The listing builds one solid part. Answer for the finished solid, in the listing's coordinates (mm). Face numbers are marked on the shaded views. A direction names the side the tool comes from. Round coordinates to 2 decimals unless told otherwise and drop trailing zeros. Loops run counter-clockwise (first coordinate to the right, second up) from the corner with the lowest first, then second, coordinate; pieces in that order, holes last. Notation, with made-up numbers: (49.25, 7) -> (94.25, 7) arc R5 ccw to (94.25, 15) -> close; hole circle Ø2 at (-38, 34). An arc over 180 degrees is marked (long way). Use a Markdown table: item, result. Add a question column.
Q1. Section C-C on y = -89 is taken. Give the vertices of the cut face in (x, z).
Q2. Section D-D on z = 46 is taken. Give the vertices of the cut face in (x, y).
Q3. For a pull along Z with two mould halves and no side action, classify the marked faces 1, 2, 3 and 4 as released by +Z, released by -Z, zero draft, split by the parting line, or undercut.
Q4. Given pin 1 Ø9.5 at (y, z) = (-19, 41) entering from +X; pin 2 Ø8 at (x, z) = (141, 8.5) entering from -Y; pin 3 Ø8 at (x, z) = (166, 42) entering from -Y, each flat-ended and moving along its own axis, determine where each tip first touches the part or whether it passes through.
Q5. Section B-B on z = 60.5 is taken. Give the vertices of the cut face in (x, y), then the cut area to 3 significant figures.
Q6. Consider line 1 (Z direction, x = 189.5, y = -5.75) (3 decimals); line 2 (Y direction, x = 177.5, z = 12.5); line 3 (X direction, y = 28.5, z = 3.5). Determine where each line is inside the solid, lowest interval first.
Q7. Section A-A on x = 189.5 is taken. Give the vertices of the cut face in (y, z) (3 decimals).
Q8. Which of the six approach directions +Z, -Z, +X, -X, +Y, -Y give full straight-line access (tool end or side, diameter ignored) to the marked faces 5, 6 and 7?
from build123d import *

# Parameters (mm, degrees)
SALIENTE_EXTRUIR1_DEPTH = 65.25
CROQUIS3_W              = 45.25
CROQUIS3_H              = 36.500322872
CORTAR_EXTRUIR1_DEPTH   = 45
CROQUIS5_R              = 2.5
CORTAR_EXTRUIR3_DEPTH   = 45
CROQUIS9_R              = 2.5
CORTAR_EXTRUIR5_DEPTH   = 45


with BuildPart() as part:
    # Croquis1 → Saliente-Extruir1 (new body)
    with BuildSketch(Plane.XY):
        with BuildLine():
            Line((209, 0), (163, 0))
            ThreePointArc((163, 0), (160.07788224, 30.725748448), (151.41629917, 60.349849592))
            Line((151.41629917, 60.349849592), (140.594792415, 60.349849592))
            ThreePointArc((140.594792415, 60.349849592), (150.24757204, -28.890605671), (108.187337522, -108.187337522))
            Line((108.187337522, -108.187337522), (115.258405333, -115.258405333))
            ThreePointArc((115.258405333, -115.258405333), (140.028326503, -83.43301371), (156.226502146, -46.500322872))
            Line((156.226502146, -46.500322872), (209, -10))
            Line((209, -10), (209, 0))
        make_face()
    extrude(amount=SALIENTE_EXTRUIR1_DEPTH)

    # Croquis3 → Cortar-Extruir1 (cut)
    with BuildSketch(Plane(origin=(209, 0, 0), x_dir=(0, 0, -1), z_dir=(1, 0, 0))):
        with Locations((-32.625, -28.250161436)):
            Rectangle(CROQUIS3_W, CROQUIS3_H)
    extrude(amount=-CORTAR_EXTRUIR1_DEPTH, mode=Mode.SUBTRACT)

    # Croquis5 → Cortar-Extruir3 (cut)
    with BuildSketch(Plane(origin=(10, 0, 0), x_dir=(0, 0, -1), z_dir=(1, 0, 0))):
        with Locations((-32.625, -172.846481178)):
            Circle(CROQUIS5_R)
    extrude(amount=-CORTAR_EXTRUIR3_DEPTH, mode=Mode.SUBTRACT)

    # Croquis9 → Cortar-Extruir5 (cut)
    with BuildSketch(Plane(origin=(0, -10, 0), x_dir=(-1, 0, 0), z_dir=(0, -1, 0))):
        with Locations((-189.5, -32.625)):
            Circle(CROQUIS9_R)
    extrude(amount=-CORTAR_EXTRUIR5_DEPTH, mode=Mode.SUBTRACT)


solid = part.part
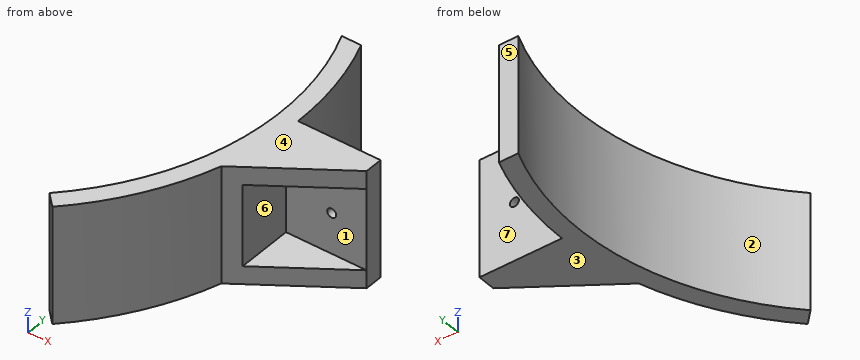
Checked values:
| question | item | result |
|---|---|---|
| 1 | outline | (124.45, 0) -> (136.56, 0) -> (136.56, 65.25) -> (124.45, 65.25) -> close |
| 2 | outline | (108.19, -108.19) -> (115.26, -115.26) arc R163 ccw to (156.23, -46.5) -> (164, -41.12) -> (164, -10) -> (209, -10) -> (209, 0) -> (163, 0) arc R163 ccw to (151.42, 60.35) -> (140.59, 60.35) arc R153 cw to start |
| 3 | face 1 | undercut |
| 3 | face 2 | zero draft |
| 3 | face 3 | released by -Z |
| 3 | face 4 | released by +Z |
| 4 | pin 1 | stops at x = 164 |
| 4 | pin 2 | stops at y = -88.32 |
| 4 | pin 3 | stops at y = -42.51 |
| 5 | outline | (108.19, -108.19) -> (115.26, -115.26) arc R163 ccw to (156.23, -46.5) -> (209, -10) -> (209, 0) -> (163, 0) arc R163 ccw to (151.42, 60.35) -> (140.59, 60.35) arc R153 cw to start |
| 5 | area | 3,140 mm2 |
| 6 | line 1 | z = 0 to 30.125, 35.125 to 65.25 |
| 6 | line 2 | y = -10 to 0 |
| 6 | line 3 | x = 150.32 to 160.49 |
| 7 | outline | (-23.487, 0) -> (0, 0) -> (0, 30.125) -> (-10, 30.125) -> (-10, 10) -> (-23.487, 10) -> close; (-23.487, 55.25) -> (-10, 55.25) -> (-10, 35.125) -> (0, 35.125) -> (0, 65.25) -> (-23.487, 65.25) -> close |
| 8 | face 5 | +Z, -Z, +X, -X, +Y |
| 8 | face 6 | +X, -Y |
| 8 | face 7 | +Z, -Z, +X, +Y |
